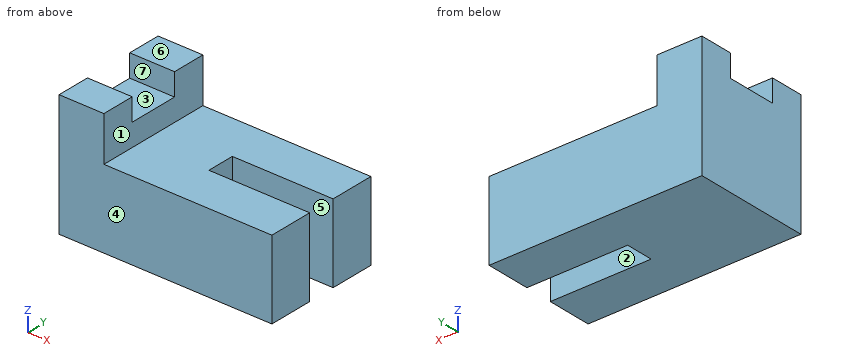
from build123d import *

# Parameters (mm, degrees)
F0_W      = 120.65
F0_H      = 66.548
F1_DEPTH  = 19.05
F2_W      = 25.4
F2_H      = 44.45
F3_DEPTH  = 66.548
F4_W      = 25.4
F4_H      = 66.548
F5_DEPTH  = 25.4
F6_W      = 25.4
F6_H      = 28.0485648255
F7_DEPTH  = 12.7
F8_W      = 25.4
F8_H      = 28.448
F9_DEPTH  = 12.7
F10_W     = 57.15
F10_H     = 15.748
F11_DEPTH = 25.4
F13_DEPTH = 25.4


with BuildPart() as f1:
    # F0 (on Top) → F1 (new body)
    with BuildSketch(Plane.XY):
        with Locations((60.325, -33.274)):
            Rectangle(F0_W, F0_H)
    extrude(amount=F1_DEPTH)

    # F2 (on face) → F3 (join)
    with BuildSketch(Plane.XZ.offset(66.548)):
        with Locations((12.7, 22.225)):
            Rectangle(F2_W, F2_H)
    extrude(amount=-F3_DEPTH)

    # F4 (on face) → F5 (join)
    with BuildSketch(Plane.XY.offset(44.45)):
        with Locations((12.7, -33.274)):
            Rectangle(F4_W, F4_H)
    extrude(amount=F5_DEPTH)

    # F6 (on face) → F7 (join)
    with BuildSketch(Plane.XY.offset(69.85)):
        with Locations((12.7, -33.4737175872)):
            Rectangle(F6_W, F6_H)
    extrude(amount=-F7_DEPTH)

    # F8 (on face) → F9 (cut)
    with BuildSketch(Plane.XY.offset(69.85)):
        with Locations((12.7, -33.274)):
            Rectangle(F8_W, F8_H)
    extrude(amount=-F9_DEPTH, mode=Mode.SUBTRACT)

    # F10 (on face) → F11 (cut)
    with BuildSketch(Plane.XY.offset(19.05)):
        with Locations((92.075, -33.274)):
            Rectangle(F10_W, F10_H)
    extrude(amount=-F11_DEPTH, mode=Mode.SUBTRACT)

    # F12 (on face) → F13 (join)
    with BuildSketch(Plane.XY.offset(19.05)):
        Polygon((88.9, 0), (25.4, 0), (25.4, -66.548), (120.65, -66.548), (120.65, -41.148), (63.5, -41.148), (63.5, -25.4), (120.65, -25.4), (120.65, 0), align=None)
    extrude(amount=F13_DEPTH)


solid = f1.part
Check sheet for the modelled part. Datum: model origin and axes. Units: mm. Face numbers are marked on the shaded views. A direction names the side the tool comes from. Give positions to 0.01 mm unless a question says otherwise; leave off trailing zeros. Loops run counter-clockwise (first coordinate to the right, second up) from the corner with the lowest first, then second, coordinate; pieces in that order, holes last. Notation, with made-up numbers: M -38.75,48 L -34.75,48 A29 ccw -34.75,84 Z; hole C -0.5,27 d1. An arc over 180 degrees is marked long. Answer as a JSON object with one key per item and string values. Group by question number.
Q1. Material ranges on line 1 along Y through (x, z) = (67.5, 10); line 2 along Z through (x, y) = (105, -15); line 3 along X through (y, z) = (-32.5, 36.5), recorded low to high. Write a range as [from, to].
Q2. Cross-section at B-B on z = 59. Record the cut outline in (x, y).
Q3. Go/stop test with flat-tipped pins: P1, Ø12.5, axis at y = -30, z = 14.5, coming from the +X side; P2, Ø8, axis at y = -46, z = 50, coming from the +X side; P3, Ø2, axis at x = 17.5, y = -43, coming from the +Z side. Record where each tip stops, or that it passes through.
Q4. Cross-section at A-A on x = 84. Record the cut outline in (y, z).
Q5. Cross-section at C-C on y = -12. Record the cut outline in (x, z), then the cut area to 3 significant figures.
Q6. Access from +Z, -Z, +X, -X, +Y, -Y to the whole of each face (thin tool, end or side, straight path). Record for the marked faces 1, 2 and 3.
Q7. Release check for a two-part mould opening along Y. For the marked faces 4, 5, 6 and 7 record: released by +Y, released by -Y, zero draft, split by the parting line, or undercut.
Q8. Cross-section at D-D on z = 50. Record the cut outline in (x, y).
Evaluation:
{
 "1": {"line 1": "y = [-66.55, -41.15], [-25.4, 0]", "line 2": "z = [0, 44.45]", "line 3": "x = [0, 63.5]"},
 "2": {"outline": "M 0,-66.55 L 25.4,-66.55 L 25.4,-47.5 L 0,-47.5 Z; M 0,-19.05 L 25.4,-19.05 L 25.4,0 L 0,0 Z"},
 "3": {"P1": "stops at x = 120.65", "P2": "stops at x = 25.4", "P3": "stops at z = 57.15"},
 "4": {"outline": "M -66.55,0 L -41.15,0 L -41.15,44.45 L -66.55,44.45 Z; M -25.4,0 L 0,0 L 0,44.45 L -25.4,44.45 Z"},
 "5": {"outline": "M 0,0 L 120.65,0 L 120.65,44.45 L 25.4,44.45 L 25.4,69.85 L 0,69.85 Z", "area": "6,010 mm2"},
 "6": {"face 1": "+Z, +X, +Y, -Y", "face 2": "+Z, -Z, +X", "face 3": "+Z, +X, -X"},
 "7": {"face 4": "released by -Y", "face 5": "undercut", "face 6": "zero draft", "face 7": "undercut"},
 "8": {"outline": "M 0,-66.55 L 25.4,-66.55 L 25.4,0 L 0,0 Z"}
}
